from build123d import *

# Parameters (mm, degrees)
F0_W     = 76.2
F0_H     = 38.1
F1_DEPTH = 25.4
F2_T     = -2.54
F4_DEPTH = 5.08


with BuildPart() as f1:
    # F0 (on Front) → F1 (new body)
    with BuildSketch(Plane.XZ):
        with Locations((38.1, 19.05)):
            Rectangle(F0_W, F0_H)
    extrude(amount=F1_DEPTH)

    # F2
    f2_openings = [f1.faces().sort_by_distance(p)[0] for p in [
        (38.1, -25.4, 19.05),
    ]]
    offset(amount=F2_T, openings=f2_openings)

    # F3 (on face) → F4 (join)
    with BuildSketch(Plane.XZ.offset(25.4)):
        Polygon((1.27, 36.83), (76.2, 36.83), (76.2, 38.1), (0, 38.1), (0, 0), (76.2, 0), (76.2, 1.27), (1.27, 1.27), align=None)
    extrude(amount=F4_DEPTH)


solid = f1.part
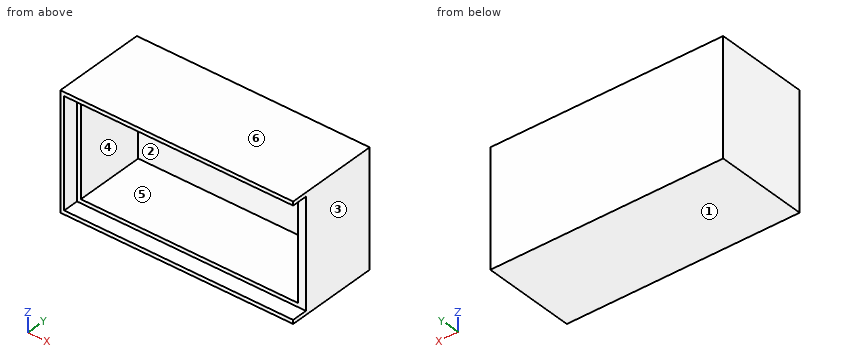
Here's how the part is built. I have some questions about the finished solid (model axes, mm). Face numbers are marked on the shaded views. A direction names the side the tool comes from. Give positions to 0.01 mm unless a question says otherwise; leave off trailing zeros. Loops run counter-clockwise (first coordinate to the right, second up) from the corner with the lowest first, then second, coordinate; pieces in that order, holes last. Notation, with made-up numbers: (51, -4.5) -> (96, -4.5) arc R19 cw to (96, 16.5) -> close; hole circle Ø1 at (81, 39). An arc over 180 degrees is marked (long way). Answer as a JSON object with one key per item and string values. Group by question number.
Item 1: Will these pins go through, and if not, where does the flat tip stop? pin 1 (2.5 mm diameter, centred on y = -27.5, z = 19.5, fed in from +X); pin 2 (10 mm diameter, centred on x = 41, z = 11.5, fed in from -Y).
Item 2: Imagine slicing it at B-B on z = 11.5. Write out the boundary of the cut face in (x, y).
Item 3: On a 3-axis mill with a long thin cutter (end or side, diameter ignored), from which of +Z, -Z, +X, -X, +Y, -Y can I reach the whole of each face in a straight line? I mean the marked faces 1 and 2. Say none if no direction works.
Item 4: I need wall thicknesses on L1, parallel to Z at x = 38.5, y = -4; L2, parallel to Z at x = 53.5, y = -26.5; L3, parallel to X at y = -14.5, z = 33. Which ranges of each line are inside material? Lowest first, please.
Item 5: Imagine slicing it at D-D on y = -27. Write out the boundary of the cut face in (x, z), then the cut area to 3 significant figures.
Item 6: Imagine slicing it at C-C on x = 50. Write out the boundary of the cut face in (y, z), then the cut area to 3 significant figures.
Item 7: Thinking about a two-plate mould opening in X: for the marked faces 3, 4, 5 and 6, which applies, pulls with the +X half, pulls with the -X half, needs draft (parallel to the pull), parting line crosses it, or undercut?
Item 8: Imagine slicing it at A-A on y = -21. Write out the boundary of the cut face in (x, z).
Answer list:
{
 "1": {"pin 1": "stops at x = 1.27", "pin 2": "stops at y = -2.54"},
 "2": {"outline": "(0, -30.48) -> (1.27, -30.48) -> (1.27, -25.4) -> (2.54, -25.4) -> (2.54, -2.54) -> (73.66, -2.54) -> (73.66, -25.4) -> (76.2, -25.4) -> (76.2, 0) -> (0, 0) -> close"},
 "3": {"face 1": "-Z, +X, -X, +Y, -Y", "face 2": "-Y"},
 "4": {"L1": "z = 0 to 2.54, 35.56 to 38.1", "L2": "z = 0 to 1.27, 36.83 to 38.1", "L3": "x = 0 to 2.54, 73.66 to 76.2"},
 "5": {"outline": "(0, 0) -> (76.2, 0) -> (76.2, 1.27) -> (1.27, 1.27) -> (1.27, 36.83) -> (76.2, 36.83) -> (76.2, 38.1) -> (0, 38.1) -> close", "area": "239 mm2"},
 "6": {"outline": "(-30.48, 0) -> (0, 0) -> (0, 38.1) -> (-30.48, 38.1) -> (-30.48, 36.83) -> (-25.4, 36.83) -> (-25.4, 35.56) -> (-2.54, 35.56) -> (-2.54, 2.54) -> (-25.4, 2.54) -> (-25.4, 1.27) -> (-30.48, 1.27) -> close", "area": "226 mm2"},
 "7": {"face 3": "pulls with the +X half", "face 4": "undercut", "face 5": "undercut", "face 6": "needs draft"},
 "8": {"outline": "(0, 0) -> (76.2, 0) -> (76.2, 38.1) -> (0, 38.1) -> close; hole (2.54, 2.54) -> (73.66, 2.54) -> (73.66, 35.56) -> (2.54, 35.56) -> close"}
}
